```python
from build123d import *

# Parameters (mm, degrees)
CROQUIS1_W              = 155
CROQUIS1_H              = 50
SALIENTE_EXTRUIR1_DEPTH = 16
CROQUIS4_W              = 22
CROQUIS4_H              = 7
SALIENTE_EXTRUIR2_DEPTH = 16
REDONDEO1_R             = 3
REDONDEO2_R             = 5
REDONDEO3_START         = 92.156121327
REDONDEO3_DEPTH         = 8.0000001
REDONDEO4_R             = 2


with BuildPart() as part:
    # Croquis1 → Saliente-Extruir1 (new body)
    with BuildSketch(Plane.XY):
        with Locations((22.656121427, -3.145967168)):
            Rectangle(CROQUIS1_W, CROQUIS1_H)
    extrude(amount=SALIENTE_EXTRUIR1_DEPTH)

    # Croquis4 → Saliente-Extruir2 (add)
    with BuildSketch(Plane.XY.offset(16)):
        with Locations((103.156121427, -31.645967168)):
            Rectangle(CROQUIS4_W, CROQUIS4_H)
    extrude(amount=-SALIENTE_EXTRUIR2_DEPTH)

    # Redondeo1
    redondeo1_edges = [part.edges().sort_by_distance(p)[0] for p in [
        (107.156121427, -28.145967168, 16),
        (107.156121427, -28.145967168, 0),
        (103.156121427, -35.145967168, 16),
        (103.156121427, -35.145967168, 0),
        (92.156121427, -35.145967168, 8),
    ]]
    fillet(redondeo1_edges, radius=REDONDEO1_R)

    # Redondeo2
    redondeo2_edges = [part.edges().sort_by_distance(p)[0] for p in [
        (-54.843878573, -3.145967168, 0),
        (-54.843878573, -3.145967168, 16),
    ]]
    fillet(redondeo2_edges, radius=REDONDEO2_R)

    # Redondeo3: read off the stored shape, not the designer's step
    # Redondeo3 outline → Redondeo3 (cut)
    with BuildSketch(Plane.YZ.offset(REDONDEO3_START)):
        with BuildLine():
            Line((-28.145967168, 13), (-28.145967168, 3))
            ThreePointArc((-28.145967168, 3), (-29.024646824, 0.878679656), (-31.145967168, 0))
            Line((-31.145967168, 0), (21.854032832, 0))
            Line((21.854032832, 0), (21.854032832, 16))
            Line((21.854032832, 16), (-31.145967168, 16))
            ThreePointArc((-31.145967168, 16), (-29.024646824, 15.121320344), (-28.145967168, 13))
        make_face()
    extrude(amount=REDONDEO3_DEPTH, mode=Mode.SUBTRACT)

    # Redondeo3 2: loft between two sections, ruled curve by curve
    redondeo3_2_from = [
        Edge.make_three_point_arc((100.156121427, 21.854032832, 8), (97.812975677, 21.854032832, 13.656854249), (92.156121427, 21.854032832, 16)),
        Edge.make_three_point_arc((100.156121427, 21.854032832, 8), (97.812975677, 21.854032832, 2.343145751), (92.156121427, 21.854032832, 0)),
        Edge.make_line((92.156121427, 21.854032832, 0), (92.156121427, 21.854032832, 16)),
    ]
    redondeo3_2_to = [
        Edge.make_three_point_arc((100.156121427, -31.145967168, 8), (97.812975677, -31.145967168, 13.656854249), (92.156121427, -31.145967168, 16)),
        Edge.make_three_point_arc((100.156121427, -31.145967168, 8), (97.812975677, -31.145967168, 2.343145751), (92.156121427, -31.145967168, 0)),
        Edge.make_line((92.156121427, -31.145967168, 0), (92.156121427, -31.145967168, 16)),
    ]
    redondeo3_2 = Solid(Shell([*[Face.make_surface_from_curves(redondeo3_2_from[k], redondeo3_2_to[k]) for k in range(3)], Face(Wire(redondeo3_2_from)), Face(Wire(redondeo3_2_to))]))
    add(redondeo3_2)

    # Redondeo4
    redondeo4_edges = [part.edges().sort_by_distance(p)[0] for p in [
        (97.812975677, 21.854032832, 13.656854249),
        (97.812975677, 21.854032832, 2.343145751),
        (-53.379412479, 21.854032832, 1.464466094),
        (-54.843878573, 21.854032832, 8),
        (-53.379412479, 21.854032832, 14.535533906),
        (-53.379412479, -28.145967168, 1.464466094),
        (-54.843878573, -28.145967168, 8),
        (-53.379412479, -28.145967168, 14.535533906),
        (21.156121377, 21.854032832, 0),
        (21.156121377, 21.854032832, 16),
        (21.156121427, -28.145967168, 0),
        (21.156121427, -28.145967168, 16),
    ]]
    fillet(redondeo4_edges, radius=REDONDEO4_R)


solid = part.part
```
The model under review builds one solid part; all positions refer to its coordinate system, in mm. A direction names the side the tool comes from. Round coordinates to 2 decimals unless told otherwise and drop trailing zeros. Order: outer loops, then holes, each group sorted by start corner. A loop starts at its lowest first (then second) coordinate and runs counter-clockwise, first axis right, second up.
Item 1: For pin 1 (1.5 mm diameter, centred on x = 56.5, z = 7.5, fed in from -Y); pin 2 (2 mm diameter, centred on y = -25, z = 10, fed in from +X); pin 3 (2 mm diameter, centred on y = -19, z = 11.5, fed in from +X), all flat-tipped, find the tip position at first contact; note any pin that passes through.
Working result:
pin 1: stops at y = -28.15
pin 2: stops at x = 100.09
pin 3: stops at x = 99.76
Item 2: Add section A-A, the plane x = 46. State the section outline as (y, z) points.
Working result:
outline: (-28.15, 2) arc R2 ccw to (-26.15, 0) - (19.85, 0) arc R2 ccw to (21.85, 2) - (21.85, 14) arc R2 ccw to (19.85, 16) - (-26.15, 16) arc R2 ccw to (-28.15, 14) - close
Item 3: To check wall thickness, follow probe 1 along Y at (x, z) = (64, 4.25); probe 2 along X at (y, z) = (14, 7.75); probe 3 along Y at (x, z) = (97, 14). State the ranges of each line that lie inside material, in increasing order.
Working result:
probe 1: y = -28.15 to 21.85
probe 2: x = -54.84 to 100.15
probe 3: y = -34.97 to 20.89
Item 4: Machinability: for faces 1 (the cylindrical face through (105.755, -29.048, 15.145)), 2 (the flat face through (105, -35.146, 8)), 3 (the cylindrical face through (105.755, -29.048, 0.855)), 4 (the flat face through (19, -28.146, 8)), 5 (the cylindrical face through (103.31, -34.29, 0.9)), which of the approach directions +Z, -Z, +X, -X, +Y, -Y give a long, thin tool a straight path to every point of the face, cutting with its end or side? Answer none if there is none.
Working result:
face 1: +Z, +X, +Y
face 2: +Z, -Z, +X, -X, -Y
face 3: -Z, +X, +Y
face 4: +Z, -Z, -X, -Y
face 5: -Z, +X, -X, -Y
